Study the drawing (mm; zero at the part's minimum x, y, z) and answer. Coordinates: 2 decimals unless noted, no trailing zeros. Order: outer loops, then holes, each group sorted by start corner. A loop starts at its lowest first (then second) coordinate and runs counter-clockwise, first axis right, second up. Notation, with made-up numbers: (-38, -21) -> (-20, -21) arc R29 cw to (-20, 1) -> close; hole circle Ø3 at (47.5, -0.5). An arc over 180 degrees is marked (long way). Put each result on its own line as item: value. Start each with the question number.
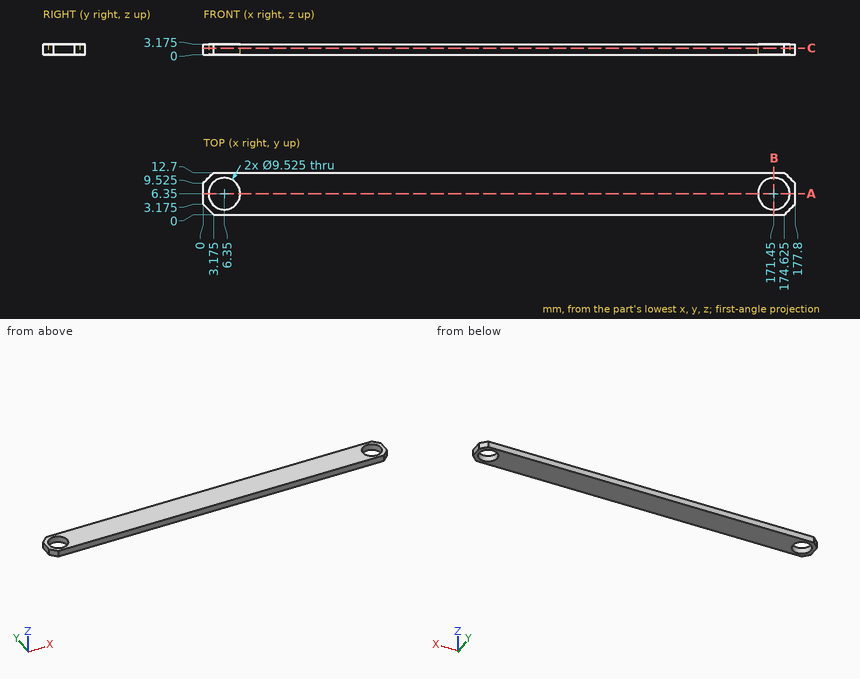
(1) Find the intervals of material crossed by L1, parallel to Y at x = 171.45, z = 1.25; L2, parallel to X at y = 9.75, z = 2.9 (3 decimals); L3, parallel to X at y = 4.25, z = 2.8, in increasing order.
(2) The part is cut by section C-C on z = 1.9. Count the separate pieces of the cut face and the enclosed holes in it, plus the area to 3 significant figures.
(3) The part is cut by section A-A on y = 6.35. Determine the outline of the cut face in (x, z) (1 decimal), plus the area to 3 significant figures.
(4) The part is cut by section B-B on x = 171.45. Determine the outline of the cut face in (y, z) (1 decimal), plus the area to 3 significant figures.
Worked out:
1. L1: 0 to 1.59, 11.11 to 12.7
1. L2: 0.225 to 3.015, 9.685 to 168.115, 174.785 to 177.575
1. L3: 0 to 2.08, 10.62 to 167.18, 175.72 to 177.8
2. separate pieces: 1
2. enclosed holes: 2
2. area: 2,100 mm2
3. outline: (0, 0) -> (1.6, 0) -> (1.6, 3.2) -> (0, 3.2) -> close; (11.1, 0) -> (166.7, 0) -> (166.7, 3.2) -> (11.1, 3.2) -> close; (176.2, 0) -> (177.8, 0) -> (177.8, 3.2) -> (176.2, 3.2) -> close
3. area: 504 mm2
4. outline: (0, 0) -> (1.6, 0) -> (1.6, 3.2) -> (0, 3.2) -> close; (11.1, 0) -> (12.7, 0) -> (12.7, 3.2) -> (11.1, 3.2) -> close
4. area: 10.1 mm2
